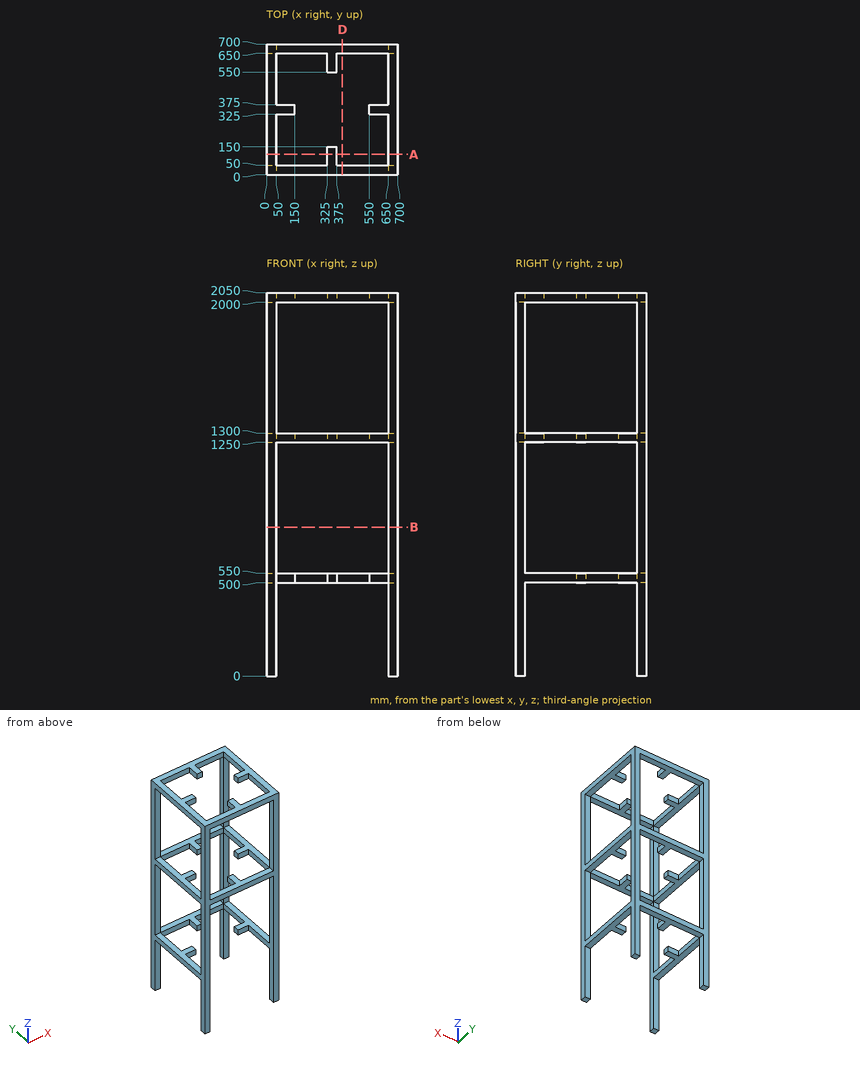
Geometry check sheet. Reference: drawing and pictorial views, mm from the part's lowest x, y, z. Coordinates: 2 decimals unless noted, no trailing zeros. Loops run counter-clockwise (first coordinate to the right, second up) from the corner with the lowest first, then second, coordinate; pieces in that order, holes last. Notation, with made-up numbers: (49.25, 66) - (100.25, 66) arc R24 cw to (100.25, 82) - close; hole circle Ø9 at (73.5, 54). An arc over 180 degrees is marked (long way). Return JSON: item names as keys, results as strings.
1. Section check B-B, the plane z = 796.5. Record the boundary of the cut face in (x, y), then the cut area to 3 significant figures.
Established:
{"outline": "(0, 0) - (50, 0) - (50, 50) - (0, 50) - close; (0, 650) - (50, 650) - (50, 700) - (0, 700) - close; (650, 0) - (700, 0) - (700, 50) - (650, 50) - close; (650, 650) - (700, 650) - (700, 700) - (650, 700) - close", "area": "10,000 mm2"}
2. Section check A-A, the plane y = 110. Count the separate pieces of the cut face and the enclosed holes in it, then the cut area to 3 significant figures.
Established:
{"separate pieces": "8", "enclosed holes": "0", "area": "20,000 mm2"}
3. Thickness scan on L1, parallel to Z at x = 276.5, y = 670; L2, parallel to Y at x = 41, z = 654.5. Record the ranges inside material, lowest first.
Established:
{"L1": "z = 500 to 550, 1250 to 1300, 2000 to 2050", "L2": "y = 0 to 50, 650 to 700"}
4. Section check D-D, the plane x = 404.5. Record the boundary of the cut face in (y, z).
Established:
{"outline": "(0, 1250) - (50, 1250) - (50, 1300) - (0, 1300) - close; (0, 2000) - (50, 2000) - (50, 2050) - (0, 2050) - close; (650, 500) - (700, 500) - (700, 550) - (650, 550) - close; (650, 1250) - (700, 1250) - (700, 1300) - (650, 1300) - close; (650, 2000) - (700, 2000) - (700, 2050) - (650, 2050) - close"}
